Work out the finished part from the listing and answer in its coordinate system (mm). Round coordinates to 2 decimals unless told otherwise and drop trailing zeros. Order: outer loops, then holes, each group sorted by start corner. A loop starts at its lowest first (then second) coordinate and runs counter-clockwise, first axis right, second up. Notation, with made-up numbers: (44, 87) - (75, 87) arc R6 cw to (75, 96) - close; hole circle Ø10 at (75.5, 43.25). An arc over 180 degrees is marked (long way). One line per question, with ' | ' between items. Start each with the question number.
from build123d import *

# Parameters (mm, degrees)
SKETCH_1_R               = 25
SKETCH_1_R_2             = 23.2
EXTRUDE_1_DEPTH          = 30
CUT_EXTRUDE_1_DEPTH      = 47.368092477
CUT_EXTRUDE_1_DEPTH_BACK = 47.368092477
FILLET_1_R               = 1


with BuildPart() as part:
    # 草图1 → 凸台-拉伸1 (new body)
    with BuildSketch(Plane.XY):
        Circle(SKETCH_1_R)
        Circle(SKETCH_1_R_2, mode=Mode.SUBTRACT)
    extrude(amount=EXTRUDE_1_DEPTH)

    # 草图3 → 切除-拉伸1 (cut, two sides: drawn at the far end of the back side and taken through both)
    with BuildSketch(Plane(origin=(0, 0, 0), x_dir=(1, 0, 0), z_dir=(0, 1, 0)).offset(-CUT_EXTRUDE_1_DEPTH_BACK)):
        with BuildLine():
            Line((-1.15, 0), (-1.15, -2.036931986))
            ThreePointArc((-1.15, -2.036931986), (0, -1.5), (1.15, -2.036931986))
            Line((1.15, -2.036931986), (1.15, 0))
            Line((1.15, 0), (-1.15, 0))
        make_face()
        with BuildLine():
            Line((-1.15, -2.036931986), (-1.15, -3.963068014))
            ThreePointArc((-1.15, -3.963068014), (0, -4.5), (1.15, -3.963068014))
            Line((1.15, -3.963068014), (1.15, -2.036931986))
            ThreePointArc((1.15, -2.036931986), (0, -1.5), (-1.15, -2.036931986))
        make_face()
        with BuildLine():
            Line((1.15, -2.036931986), (1.15, -3.963068014))
            ThreePointArc((1.15, -3.963068014), (1.409787218, -3.512347538), (1.5, -3))
            ThreePointArc((1.5, -3), (1.409787218, -2.487652462), (1.15, -2.036931986))
        make_face()
        with BuildLine():
            ThreePointArc((-1.15, -2.036931986), (-1.5, -3), (-1.15, -3.963068014))
            Line((-1.15, -3.963068014), (-1.15, -2.036931986))
        make_face()
    extrude(amount=CUT_EXTRUDE_1_DEPTH + CUT_EXTRUDE_1_DEPTH_BACK, mode=Mode.SUBTRACT)

    # 圆角1
    fillet_1_edges = [part.edges().sort_by_distance(p)[0] for p in [
        (-1.15, 24.072508154, 0),
        (-1.15, -24.072508154, 0),
        (1.15, -24.072508154, 0),
        (1.15, 24.072508154, 0),
    ]]
    fillet(fillet_1_edges, radius=FILLET_1_R)


solid = part.part
1) Section A-A on x = 0 is taken. Give the vertices of the cut face in (y, z), and give its area (3 significant figures).
2) Flat-ended cylindrical pins translate along their axes: pin 1 (2 mm diameter, centred on x = -6, z = 7.5, fed in from +Y); pin 2 (4 mm diameter, centred on x = -11.5, z = 23.5, fed in from -Y); pin 3 (10 mm diameter, centred on y = -16, z = 5.5, fed in from +X). Find the tip coordinate at first contact, or state that the pin passes through.
3) Determine the mould class of faces 1 (the flat face through (17, -17, 30)), 2 (the cylindrical face through (-23.178, 1.02, 14.79)), 3 (the cylindrical face through (23.846, 7.509, 14.79)) for opening direction X: released by +X, released by -X, zero draft, split by the parting line, or undercut.
4) Section C-C on z = 22 is taken. Give the vertices of the cut face in (x, y), and give its area (3 significant figures).
5) Section B-B on y = 0 is taken. Give the vertices of the cut face in (x, z).
6) Straight lines are drawn through the part: line 1 (Y direction, x = 0, z = 15); line 2 (X direction, y = -13, z = 6). For each, find the intervals that lie inside material, in ascending order.
Recorded:
1) outline: (-25, 4.5) - (-23.2, 4.5) - (-23.2, 30) - (-25, 30) - close; (23.2, 4.5) - (25, 4.5) - (25, 30) - (23.2, 30) - close | area: 91.8 mm²
2) pin 1: stops at y = 24.49 | pin 2: stops at y = -23.12 | pin 3: stops at x = 22.45
3) face 1: zero draft | face 2: undercut | face 3: split by the parting line
4) outline: circle Ø50 at (0, 0); hole circle Ø46.4 at (0, 0) | area: 273 mm²
5) outline: (-25, 0) - (-23.2, 0) - (-23.2, 30) - (-25, 30) - close; (23.2, 0) - (25, 0) - (25, 30) - (23.2, 30) - close
6) line 1: y = -25 to -23.2, 23.2 to 25 | line 2: x = -21.35 to -19.22, 19.22 to 21.35
